Source: CAD feature listing. Evaluate the final solid. Frame: model axes, mm. Face numbers are marked on the shaded views. Round coordinates to 2 decimals unless told otherwise and drop trailing zeros. Order: outer loops, then holes, each group sorted by start corner. A loop starts at its lowest first (then second) coordinate and runs counter-clockwise, first axis right, second up. Notation, with made-up numbers: M -40,60.25 L 6,60.25 A21 ccw 6,99.25 Z; hole C 55.5,18 d6. An arc over 180 degrees is marked long. Use one line per item in the form item = value. Start each with the question number.
Q1. Section B-B (y = 26.5). Return the cut outline in (x, z).
Q2. Material intervals for probe 1 along X at (y, z) = (36.4, 4); probe 2 along Y at (x, z) = (-123, 4.5); probe 3 along X at (y, z) = (17.5, 7.75), sorted ascending.
Q3. Section C-C (z = 6.75). Return the cut outline in (x, y).
Q4. Section A-A (x = -147). Return the cut outline in (y, z).
Q5. Contact query for a flat-ended pin moving along its axis: pin 1 (2 mm diameter, centred on x = -128.82, z = 4, fed in from +Y). Output: stop coordinate, or through.
Q6. Section D-D (y = 19.5). Return the cut outline in (x, z).
Q7. Pull-direction query (Y, two-part tool) for the marked faces 1, 2 and 3; classes: pulls with the +Y half, pulls with the -Y half, needs draft (parallel to the pull), parting line crosses it, or undercut.
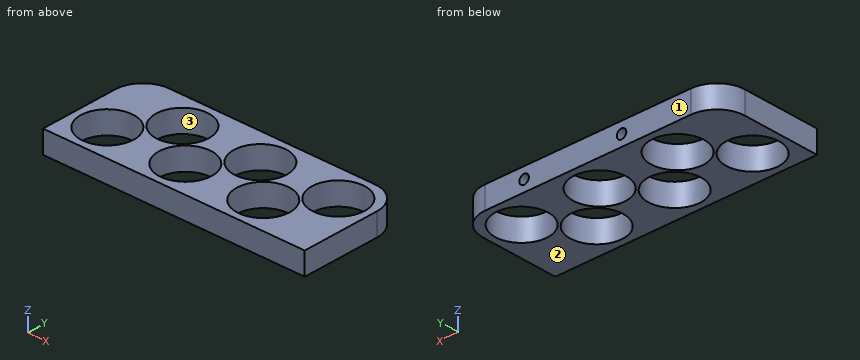
from build123d import *

# Parameters (mm, degrees)
SKETCH2_W           = 94
SKETCH2_H           = 38
SKETCH2_R           = 9.5
BOSS_EXTRUDE1_DEPTH = 8
FILLET1_R           = 10
SKETCH3_R           = 1.7
CUT_EXTRUDE1_DEPTH  = 5


with BuildPart() as part:
    # Sketch2 → Boss-Extrude1 (new body)
    with BuildSketch(Plane.XY):
        with Locations((-151.821569614, 20.991771931)):
            Rectangle(SKETCH2_W, SKETCH2_H)
        with Locations((-186.821569614, 13.991771931)):
            Circle(SKETCH2_R, mode=Mode.SUBTRACT)
        with Locations((-158.821569614, 13.991771931)):
            Circle(SKETCH2_R, mode=Mode.SUBTRACT)
        with Locations((-130.821569614, 13.991771931)):
            Circle(SKETCH2_R, mode=Mode.SUBTRACT)
        with Locations((-144.821569614, 27.991771931)):
            Circle(SKETCH2_R, mode=Mode.SUBTRACT)
        with Locations((-116.821569614, 27.991771931)):
            Circle(SKETCH2_R, mode=Mode.SUBTRACT)
        with Locations((-172.821569614, 27.991771931)):
            Circle(SKETCH2_R, mode=Mode.SUBTRACT)
    extrude(amount=BOSS_EXTRUDE1_DEPTH)

    # Fillet1
    fillet1_edges = [part.edges().sort_by_distance(p)[0] for p in [
        (-198.821569614, 39.991771931, 4),
        (-104.821569614, 39.991771931, 4),
    ]]
    fillet(fillet1_edges, radius=FILLET1_R)

    # Sketch3 → Cut-Extrude1 (cut)
    with BuildSketch(Plane(origin=(0, 39.991771931, 0), x_dir=(1, 0, 0), z_dir=(0, 1, 0))):
        with Locations((-163.821569614, -4)):
            Circle(SKETCH3_R)
        with Locations((-128.821569614, -4)):
            Circle(SKETCH3_R)
    extrude(amount=-CUT_EXTRUDE1_DEPTH, mode=Mode.SUBTRACT)


solid = part.part
Results list:
q1.outline = M -198.82,0 L -182.2,0 L -182.2,8 L -198.82,8 Z; M -163.44,0 L -154.2,0 L -154.2,8 L -163.44,8 Z; M -135.44,0 L -126.2,0 L -126.2,8 L -135.44,8 Z; M -107.44,0 L -104.82,0 L -104.82,8 L -107.44,8 Z
q2.probe_1 = -196.5 to -177.24, -168.4 to -165.52, -162.12 to -149.24, -140.4 to -130.52, -127.12 to -121.24, -112.4 to -107.14
q2.probe_2 = 1.99 to 8.6, 19.38 to 20.78, 35.21 to 39.99
q2.probe_3 = -198.82 to -195.65, -177.99 to -167.65, -149.99 to -139.65, -121.99 to -104.82
q3.outline = M -198.82,1.99 L -104.82,1.99 L -104.82,29.99 A10 ccw -114.82,39.99 L -188.82,39.99 A10 ccw -198.82,29.99 Z; hole C -186.82,13.99 d19; hole C -172.82,27.99 d19; hole C -158.82,13.99 d19; hole C -144.82,27.99 d19; hole C -130.82,13.99 d19; hole C -116.82,27.99 d19
q4.outline = M 1.99,0 L 18.74,0 L 18.74,8 L 1.99,8 Z; M 37.24,0 L 39.99,0 L 39.99,8 L 37.24,8 Z
q5.pin_1 = 34.99
q6.outline = M -198.82,0 L -194.56,0 L -194.56,8 L -198.82,8 Z; M -179.08,0 L -177.08,0 L -177.08,8 L -179.08,8 Z; M -168.56,0 L -166.56,0 L -166.56,8 L -168.56,8 Z; M -151.08,0 L -149.08,0 L -149.08,8 L -151.08,8 Z; M -140.56,0 L -138.56,0 L -138.56,8 L -140.56,8 Z; M -123.08,0 L -121.08,0 L -121.08,8 L -123.08,8 Z; M -112.56,0 L -104.82,0 L -104.82,8 L -112.56,8 Z
q7.face_1 = pulls with the +Y half
q7.face_2 = needs draft
q7.face_3 = undercut
